Geometry: final body of the model. Coordinates: model frame, mm. Face numbers are marked on the shaded views. Round coordinates to 2 decimals unless told otherwise and drop trailing zeros. Write each loop counter-clockwise with the first axis right and the second up, starting at its lowest first coordinate (ties: lowest second). Pieces come first, ordered by that corner, then holes. Notation, with made-up numbers: (-11.5, 31) -> (5.5, 31) arc R11 cw to (5.5, 47) -> close; hole circle Ø7 at (48, -36). An arc over 180 degrees is marked (long way). One line per item, written item: value. Start each with the question number.
from build123d import *

# Parameters (mm, degrees)
SKETCH_W        = 34
SKETCH_H        = 34
PAD_DEPTH       = 80
POCKET_DEPTH    = 80
SKETCH002_R     = 3
POCKET001_DEPTH = 4
SKETCH003_R     = 3
POCKET002_DEPTH = 4
SKETCH004_R     = 4
POCKET003_DEPTH = 2
SKETCH005_R     = 4
POCKET004_DEPTH = 2
SKETCH006_W     = 6.4
SKETCH006_H     = 3
SKETCH006_W_2   = 8
SKETCH006_H_2   = 8
POCKET005_DEPTH = 12


with BuildPart() as part:
    # Sketch → Pad (new body)
    with BuildSketch(Plane.XY):
        with Locations((17, 17)):
            Rectangle(SKETCH_W, SKETCH_H)
    extrude(amount=PAD_DEPTH)

    # Sketch001 (on Face6 of Pad) → Pocket (cut)
    with BuildSketch(Plane.XY.offset(80)):
        Polygon((6.5, 27.5), (14, 27.5), (14, 23.5), (17, 21), (20, 23.5), (20, 27.5), (27.5, 27.5), (27.5, 19.5), (23.5, 19.5), (21, 17), (23.5, 14), (27.5, 14), (27.5, 6.5), (20, 6.5), (20, 10.5), (17, 13), (14, 10.5), (14, 6.5), (6.5, 6.5), (6.5, 14), (10.5, 14), (13, 17), (10.5, 19.5), (6.5, 19.5), align=None)
    extrude(amount=-POCKET_DEPTH, mode=Mode.SUBTRACT)

    # Sketch002 (on Face2 of Pocket) → Pocket001 (cut)
    with BuildSketch(Plane(origin=(0, 0, 0), x_dir=(0, -1, 0), z_dir=(-1, 0, 0))):
        with Locations((-17, 60)):
            Circle(SKETCH002_R)
        with Locations((-17, 20)):
            Circle(SKETCH002_R)
    extrude(amount=-POCKET001_DEPTH, mode=Mode.SUBTRACT)

    # Sketch003 (on Face3 of Pocket001) → Pocket002 (cut)
    with BuildSketch(Plane.YZ.offset(34)):
        with Locations((17, 60)):
            Circle(SKETCH003_R)
        with Locations((17, 20)):
            Circle(SKETCH003_R)
    extrude(amount=-POCKET002_DEPTH, mode=Mode.SUBTRACT)

    # Sketch004 (on Face1 of Pocket002) → Pocket003 (cut)
    with BuildSketch(Plane(origin=(0, 34, 0), x_dir=(-1, 0, 0), z_dir=(0, 1, 0))):
        with Locations((-27, 60)):
            Circle(SKETCH004_R)
        with Locations((-7, 60)):
            Circle(SKETCH004_R)
        with Locations((-27, 20)):
            Circle(SKETCH004_R)
        with Locations((-7, 20)):
            Circle(SKETCH004_R)
    extrude(amount=-POCKET003_DEPTH, mode=Mode.SUBTRACT)

    # Sketch005 (on Face10 of Pocket003) → Pocket004 (cut)
    with BuildSketch(Plane.XZ):
        with Locations((7, 60)):
            Circle(SKETCH005_R)
        with Locations((27, 60)):
            Circle(SKETCH005_R)
        with Locations((7, 20)):
            Circle(SKETCH005_R)
        with Locations((27, 20)):
            Circle(SKETCH005_R)
    extrude(amount=-POCKET004_DEPTH, mode=Mode.SUBTRACT)

    # Sketch006 (on Face4 of Pocket004) → Pocket005 (cut)
    with BuildSketch(Plane.XY.offset(80)):
        with Locations((17, 1.5)):
            Rectangle(SKETCH006_W, SKETCH006_H)
        with Locations((17, 10.5)):
            Rectangle(SKETCH006_W_2, SKETCH006_H_2)
    extrude(amount=-POCKET005_DEPTH, mode=Mode.SUBTRACT)


solid = part.part
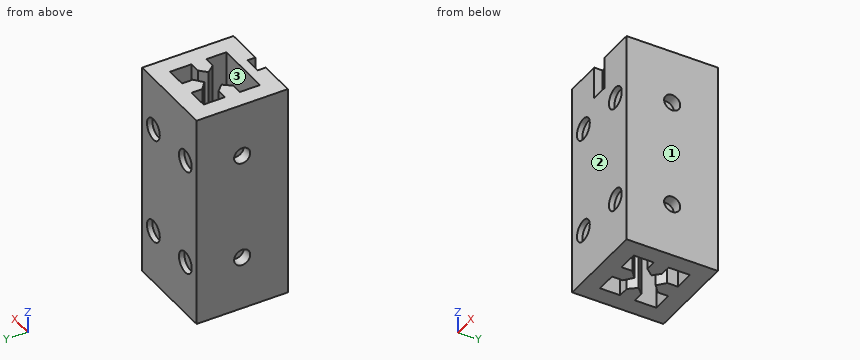
(1) Line query: probe 1 along Z at (x, y) = (31.9, 17); probe 2 along Z at (x, y) = (27, 33.35); probe 3 along Y at (x, z) = (26, 5.5). Output: solid intervals per line, ascending.
(2) Pin query (flat end, axial travel): pin 1 (8 mm diameter, centred on x = 22.5, z = 14, fed in from -Y); pin 2 (1.8 mm diameter, centred on y = 18.5, z = 20, fed in from -X); pin 3 (3 mm diameter, centred on x = 26.5, z = 60, fed in from +Y); pin 4 (6.5 mm diameter, centred on x = 17.5, y = 10, fed in from +Z). Return the tip coordinate at first contact, or that it passes through.
(3) Section query D-D (y = 9.5). Output: boundary loops of the cut face in (x, z), and give its area (3 significant figures).
(4) Section query C-C (x = 19). Output: boundary loops of the cut face in (y, z), and give its area (3 significant figures).
(5) Section query A-A (y = 26). Output: boundary loops of the cut face in (x, z).
(6) Pull-direction query (Y, two-part tool) for the marked faces 1, 2 and 3; classes: pulls with the +Y half, pulls with the -Y half, needs draft (parallel to the pull), parting line crosses it, or undercut.
(7) Section query B-B (z = 11). Output: boundary loops of the cut face in (x, y).
Results list:
1. probe 1: z = 0 to 17, 23 to 57, 63 to 80
1. probe 2: z = 0 to 16, 24 to 56, 64 to 80
1. probe 3: y = 0 to 6.5, 14 to 19.5, 27.5 to 34
2. pin 1: stops at y = 0
2. pin 2: stops at x = 4
2. pin 3: stops at y = 32
2. pin 4: stops at z = 68
3. outline: (0, 0) -> (6.5, 0) -> (6.5, 80) -> (0, 80) -> close; (14, 0) -> (20, 0) -> (20, 68) -> (14, 68) -> close; (27.5, 0) -> (34, 0) -> (34, 80) -> (27.5, 80) -> close
3. area: 1,450 mm^2
4. outline: (0, 0) -> (11.33, 0) -> (11.33, 68) -> (6.5, 68) -> (6.5, 80) -> (3, 80) -> (3, 68) -> (0, 68) -> close; (22.67, 0) -> (34, 0) -> (34, 80) -> (22.67, 80) -> close
4. area: 1,720 mm^2
5. outline: (0, 0) -> (6.5, 0) -> (6.5, 80) -> (0, 80) -> close; (14, 0) -> (20, 0) -> (20, 80) -> (14, 80) -> close; (27.5, 0) -> (34, 0) -> (34, 80) -> (27.5, 80) -> close
6. face 1: needs draft
6. face 2: pulls with the -Y half
6. face 3: undercut
7. outline: (0, 0) -> (34, 0) -> (34, 34) -> (0, 34) -> close; hole (6.5, 6.5) -> (14, 6.5) -> (14, 10.5) -> (17, 13) -> (20, 10.5) -> (20, 6.5) -> (27.5, 6.5) -> (27.5, 14) -> (23.5, 14) -> (21, 17) -> (23.5, 19.5) -> (27.5, 19.5) -> (27.5, 27.5) -> (20, 27.5) -> (20, 23.5) -> (17, 21) -> (14, 23.5) -> (14, 27.5) -> (6.5, 27.5) -> (6.5, 19.5) -> (10.5, 19.5) -> (13, 17) -> (10.5, 14) -> (6.5, 14) -> close
